Autodesk Fusion 360 part; units mm, degrees
sketch "Sketch1" plane through (0, 0, 0) normal (0, 0, 1) x (1, 0, 0)
  circle A0 centre (0, 0) radius 4.75
  dimension "d1" = 9.5
extrude "Extrude1" add sketch "Sketch1" along normal blind 35
sketch "Sketch2" plane through (0, 0, 35) normal (0, 0, 1) x (-1, 0, 0)
  circle A0 centre (0, 0) radius 4.75
  arc A1 (-1, -1.118) -> (-1, 1.118) centre (0, 0) ccw
  line L0 (-1, -1.118) -> (-1, 1.118)
extrude "Extrude2" cut sketch "Sketch2" against normal blind 12 contours A1 L0
sketch "Sketch3" plane through (0, 0, 0) normal (0, 0, -1) x (1, 0, 0)
  circle A0 centre (0, 0) radius 4.75
  line L0 (2.75, 1.25) -> (-2.75, 1.25)
  line L1 (-2.75, 1.25) -> (-2.75, -1.25)
  line L2 (-2.75, -1.25) -> (2.75, -1.25)
  line L3 (2.75, -1.25) -> (2.75, 1.25)
  dimension "d9" = 5.5
  dimension "d10" = 2.5
extrude "Extrude3" cut sketch "Sketch3" against normal blind 18 contours L0 L1 L2 L3
extrude "Extrude4" cut 1 faces at (-0.9167, -0.4167, 18) along direction (0, 0, 1) blind 4
extrude "Extrude5" cut 1 faces at (0.1183, 2.4122, 0) along direction (0, 0, 1) blind 5
extrude "Extrude6" cut 1 faces at (0.1183, 2.4122, 5) along direction (0, 0, 1) blind 1
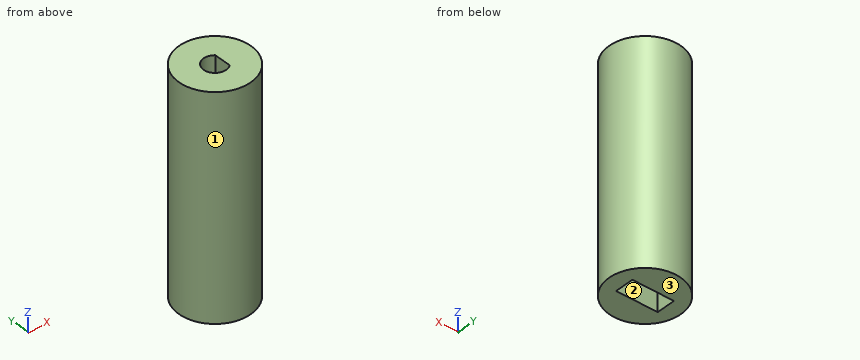
Part model, mm, in its own coordinate system. Face numbers are marked on the shaded views. Round coordinates to 2 decimals unless told otherwise and drop trailing zeros. Write each loop counter-clockwise with the first axis right and the second up, starting at its lowest first coordinate (ties: lowest second). Pieces come first, ordered by that corner, then holes.
Item 1: Two-plate mould, pull along X, no slides. Class the marked faces 1, 2 and 3: +X half, -X half, draft (parallel to the pull), parting line (faces both ways), or undercut.
Results:
face 1: parting line
face 2: undercut
face 3: draft
Item 2: Drop a flat-ended pin along its axis: pin 1 Ø5 at (x, z) = (4, 28) entering from -Y. Give the stop position or say it passes through.
Results:
pin 1: stops at y = -4.51
Item 3: Cut at C-C, the plane z = 25.5. Give the cut face in (x, y).
Results:
outline: circle Ø9.5 at (0, 0); hole (1, -1.12) - (1, 1.12) arc R1.5 ccw (long way) to start
Item 4: Cut at B-B, the plane y = 0.75. Give the cut face in (x, z).
Results:
outline: (-4.69, 6) - (-2.75, 6) - (-2.75, 22) - (2.75, 22) - (2.75, 6) - (4.69, 6) - (4.69, 35) - (1, 35) - (1, 23) - (-1.3, 23) - (-1.3, 35) - (-4.69, 35) - close
Item 5: Probe L1, parallel to Y at x = 0, z = 30.5; L2, parallel to X at y = -1, z = 17.5; L3, parallel to Y at x = -1.5, z = 21.5. List the from-to ranges inside material, lowest first.
Results:
L1: y = -4.75 to -1.5, 1.5 to 4.75
L2: x = -4.64 to -2.75, 2.75 to 4.64
L3: y = -4.51 to -1.25, 1.25 to 4.51
Item 6: Cut at A-A, the plane x = 0. Give the cut face in (y, z).
Results:
outline: (-4.75, 6) - (-1.25, 6) - (-1.25, 22) - (1.25, 22) - (1.25, 6) - (4.75, 6) - (4.75, 35) - (1.5, 35) - (1.5, 23) - (-1.5, 23) - (-1.5, 35) - (-4.75, 35) - close
Item 7: Cut at D-D, the plane x = 2. Give the cut face in (y, z), plus the area to 3 significant figures.
Results:
outline: (-4.31, 6) - (-1.25, 6) - (-1.25, 22) - (1.25, 22) - (1.25, 6) - (4.31, 6) - (4.31, 35) - (-4.31, 35) - close
area: 210 mm2
